```python
from build123d import *

# Parameters (mm, degrees)
SKETCH1_R                = 1.5625
BOSS_EXTRUDE1_DEPTH      = 3
SKETCH2_R                = 1.96
BOSS_EXTRUDE2_DEPTH      = 4
BOSS_EXTRUDE2_DEPTH_BACK = 3
CUT_EXTRUDE1_DEPTH       = 11.5
CHAMFER1_SIZE            = 0.5
CUT_EXTRUDE3_DEPTH       = 4.7625
FILLET1_R                = 6
SKETCH6_R                = 2
SKETCH6_R_2              = 1.25
CUT_EXTRUDE4_DEPTH       = 1.25


with BuildPart() as part:
    # Sketch1 → Boss-Extrude1 (new body)
    with BuildSketch(Plane(origin=(0, 0, 0), x_dir=(1, 0, 0), z_dir=(0, 1, 0))):
        with BuildLine():
            Line((3.181980515, -15.181980515), (18.5, 0.136038969))
            Line((18.5, 0.136038969), (18.5, 8))
            ThreePointArc((18.5, 8), (17.181980515, 11.181980515), (14, 12.5))
            Line((14, 12.5), (6, 12.5))
            Line((6, 12.5), (1, 7.5))
            Line((1, 7.5), (-4.5, 2))
            Line((-4.5, 2), (-4.5, -6.5))
            Line((-4.5, -6.5), (-4.5, -12))
            ThreePointArc((-4.5, -12), (-1.722075446, -16.157457896), (3.181980515, -15.181980515))
        make_face()
        with Locations((0, -12)):
            Circle(SKETCH1_R, mode=Mode.SUBTRACT)
        with Locations((14, 8)):
            Circle(SKETCH1_R, mode=Mode.SUBTRACT)
    extrude(amount=BOSS_EXTRUDE1_DEPTH)

    # Sketch2 → Boss-Extrude2 (add, two sides)
    with BuildSketch(Plane.XZ) as boss_extrude2_sk:
        Polygon((9, -9), (5, -9), (5, -8), (-4.5, -8), (-4.5, 8), (5, 8), (5, 9), (9, 9), align=None)
        Circle(SKETCH2_R, mode=Mode.SUBTRACT)
    extrude(amount=BOSS_EXTRUDE2_DEPTH)
    extrude(boss_extrude2_sk.sketch, amount=-BOSS_EXTRUDE2_DEPTH_BACK)

    # Sketch3 → Cut-Extrude1 (cut)
    with BuildSketch(Plane.ZY.offset(4.5)):
        with BuildLine():
            Line((-4.921188881, -1.62), (4.921188881, -1.62))
            ThreePointArc((4.921188881, -1.62), (6.276166224, 0.515601174), (6.75, 3))
            Line((6.75, 3), (-6.75, 3))
            ThreePointArc((-6.75, 3), (-6.276166224, 0.515601174), (-4.921188881, -1.62))
        make_face()
    extrude(amount=-CUT_EXTRUDE1_DEPTH, mode=Mode.SUBTRACT)

    # Chamfer1
    chamfer1_edges = [part.edges().sort_by_distance(p)[0] for p in [
        (9, -2, 9),
        (9, -2, -9),
        (7, -1.62, 0),
        (7, 0.515601174, -6.276166224),
        (7, 0.515601174, 6.276166224),
    ]]
    chamfer(chamfer1_edges, length=CHAMFER1_SIZE)

    # Sketch5 → Cut-Extrude3 (cut)
    with BuildSketch(Plane(origin=(0, 0, -8), x_dir=(-1, 0, 0), z_dir=(0, 0, -1))):
        Polygon((4.5, -1.62), (-0.12, 3), (4.5, 3), align=None)
    extrude(amount=-CUT_EXTRUDE3_DEPTH, mode=Mode.SUBTRACT)

    # Fillet1
    fillet1_edges = [part.edges().sort_by_distance(p)[0] for p in [
        (18.5, 1.5, -0.136038969),
    ]]
    fillet(fillet1_edges, radius=FILLET1_R)

    # Sketch6 → Cut-Extrude4 (cut)
    with BuildSketch(Plane(origin=(0, 3, 0), x_dir=(1, 0, 0), z_dir=(0, 1, 0))):
        with Locations((11.5, 0)):
            Circle(SKETCH6_R)
        with Locations((4.5, -9.75)):
            Circle(SKETCH6_R_2)
        with Locations((7.5, 9.5)):
            Circle(SKETCH6_R_2)
    extrude(amount=-CUT_EXTRUDE4_DEPTH, mode=Mode.SUBTRACT)


solid = part.part
```
Work out the finished part from the listing and answer in its coordinate system (mm). A direction names the side the tool comes from. Round coordinates to 2 decimals unless told otherwise and drop trailing zeros. Write each loop counter-clockwise with the first axis right and the second up, starting at its lowest first coordinate (ties: lowest second). Pieces come first, ordered by that corner, then holes. Notation, with made-up numbers: (14.25, 45.5) -> (57.25, 45.5) arc R27 cw to (57.25, 61.5) -> close; hole circle Ø7 at (-21, -39.75). An arc over 180 degrees is marked (long way). Write each question's results on one line, items separated by ' | '.
Q1. Straight lines are drawn through the part: line 1 along X through (y, z) = (2, -4.5); line 2 along Y through (x, z) = (13.75, 1); line 3 along Y through (x, z) = (-2.25, 4.25). For each, find the intervals that lie inside material, in ascending order. Write a range as [from, to].
Data:
line 1: [7, 18.5] | line 2: [0, 3] | line 3: [-4, -1.62]
Q2. Determine the mould class of faces 1 (the cylindrical face through (18.03, 1.52, -0.29)), 2 (the flat face through (7, 1, 0)), 3 (the cylindrical face through (15.49, 1.48, -8.47)) for opening direction X: released by +X, released by -X, zero draft, split by the parting line, or undercut.
Data:
face 1: released by +X | face 2: released by -X | face 3: undercut
Q3. Which of the six approach directions +Z, -Z, +X, -X, +Y, -Y give full straight-line access (tool end or side, diameter ignored) to faces 4 (the flat face through (0, -1, -8)), 5 (the flat face through (4, 1.75, 10)), 6 (the flat face through (-2.74, 0.14, -7.17)), 7 (the flat face through (7, -2, -9)), 8 (the conical face through (6.8, 0.66, -6.01))?
Data:
face 4: -Z, -X, -Y | face 5: +Y | face 6: -Z, -X, +Y | face 7: -Z, +X, -X, -Y | face 8: -X, +Y
Q4. Section B-B, the plane x = -0.25 is taken. Write down the section's boundary in (y, z).
Data:
outline: (-4, -8) -> (2.63, -8) -> (2.63, -6.74) arc R6.75 cw to (-1.62, -4.92) -> (-1.62, -1.94) -> (-4, -1.94) -> close; (-4, 1.94) -> (-1.62, 1.94) -> (-1.62, 4.92) arc R6.75 cw to (3, 6.75) -> (3, 10.46) -> (0, 10.46) -> (0, 8) -> (-4, 8) -> close; (0, 13.54) -> (3, 13.54) -> (3, 16.49) -> (0, 16.49) -> close
Q5. Flat-ended cylindrical pins translate along their axes: P1, Ø4, axis at y = -3, z = -9, coming from the +X side; P2, Ø1.5, axis at x = 10.5, z = 10.5, coming from the +Y side; P3, Ø1.8, axis at x = 7.5, y = -2.5, coming from the +Z side; P4, Ø1.1, axis at y = -2.5, z = -8.5, coming from the -X side. Find the tip coordinate at first contact, or state that the pin passes through.
Data:
P1: x = 9 | P2: through | P3: z = 9 | P4: x = -4.5
Q6. Section A-A, the plane y = -2.75 is taken. Write down the section's boundary in (x, z).
Data:
outline: (-4.5, -8) -> (5, -8) -> (5, -9) -> (8.5, -9) -> (9, -8.5) -> (9, 8.5) -> (8.5, 9) -> (5, 9) -> (5, 8) -> (-4.5, 8) -> close; hole circle Ø3.92 at (0, 0)
Q7. Section D-D, the plane x = 11.5 is taken. Write down the section's boundary in (y, z), then the cut area to 3 significant figures.
Data:
outline: (0, -12.5) -> (3, -12.5) -> (3, -2) -> (1.75, -2) -> (1.75, 2) -> (3, 2) -> (3, 6.86) -> (0, 6.86) -> close | area: 53.1 mm^2
Q8. Section C-C, the plane z = 0 is taken. Write down the section's boundary in (x, y).
Data:
outline: (-4.5, -4) -> (-1.96, -4) -> (-1.96, -1.62) -> (-4.5, -1.62) -> close; (1.96, -4) -> (9, -4) -> (9, 0) -> (17.9, 0) -> (17.9, 3) -> (13.5, 3) -> (13.5, 1.75) -> (9.5, 1.75) -> (9.5, 3) -> (7, 3) -> (7, -1.12) -> (6.5, -1.62) -> (1.96, -1.62) -> close
